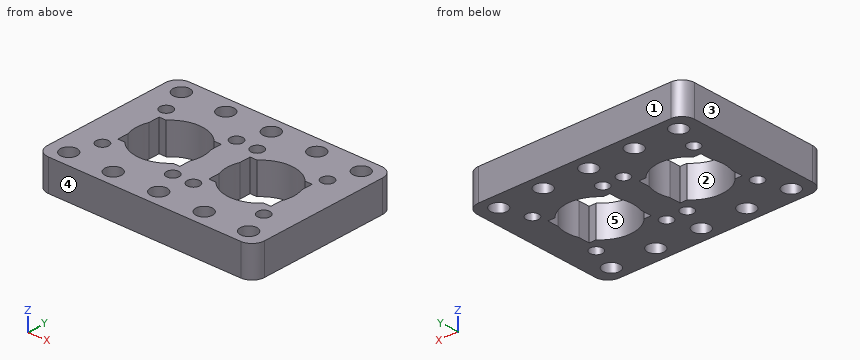
Autodesk Inventor part; units mm, degrees
ref_plane "YZ Plane" through (0, 0, 0) normal (1, 0, 0) x (0, 1, 0)
ref_plane "XZ Plane" through (0, 0, 0) normal (0, 1, 0) x (-1, 0, 0)
ref_plane "XY Plane" through (0, 0, 0) normal (0, 0, 1) x (1, 0, 0)
sketch "Sketch1" plane through (0, 0, 0) normal (0, 0, 1) x (1, 0, 0)
  line L0 (-22, 0) -> (22, 0) construction
  circle A0 centre (-22, 0) radius 16
  circle A1 centre (22, 0) radius 16
  line L1 (43.5, -30) -> (-43.5, -30) construction
  line L2 (-43.5, -30) -> (-43.5, 30) construction
  line L3 (-43.5, 30) -> (43.5, 30) construction
  line L4 (43.5, 30) -> (43.5, -30) construction
  line L5 (43.5, -30) -> (-43.5, 30) construction
  line L6 (-43.5, -30) -> (43.5, 30) construction
  circle A2 centre (-43.5, 30) radius 4
  circle A3 centre (0, 30) radius 4
  circle A4 centre (43.5, 30) radius 4
  circle A5 centre (43.5, -30) radius 4
  circle A6 centre (-43.5, -30) radius 4
  circle A7 centre (0, -30) radius 4
  line L7 (-52.5, -37.5) -> (52.5, -37.5)
  line L8 (52.5, -37.5) -> (52.5, 37.5)
  line L9 (52.5, 37.5) -> (-52.5, 37.5)
  line L10 (-52.5, 37.5) -> (-52.5, -37.5)
  line L11 (-52.5, -37.5) -> (52.5, 37.5) construction
  line L12 (52.5, -37.5) -> (-52.5, 37.5) construction
  line L13 (-5, -17) -> (-39, -17) construction
  line L14 (-39, -17) -> (-39, 17) construction
  line L15 (-39, 17) -> (-5, 17) construction
  line L16 (-5, 17) -> (-5, -17) construction
  line L17 (-5, -17) -> (-39, 17) construction
  line L18 (-39, -17) -> (-5, 17) construction
  line L19 (39, -17) -> (5, -17) construction
  line L20 (5, -17) -> (5, 17) construction
  line L21 (5, 17) -> (39, 17) construction
  line L22 (39, 17) -> (39, -17) construction
  line L23 (39, -17) -> (5, 17) construction
  line L24 (5, -17) -> (39, 17) construction
  circle A8 centre (-39, 17) radius 3
  circle A9 centre (-39, -17) radius 3
  circle A10 centre (-5, -17) radius 3
  circle A11 centre (-5, 17) radius 3
  circle A12 centre (5, 17) radius 3
  circle A13 centre (5, -17) radius 3
  circle A14 centre (39, -17) radius 3
  circle A15 centre (39, 17) radius 3
  point P0 (0, 0)
  point P1 (0, 0)
  dimension "d0" = 60
  dimension "d1" = 87
  dimension "d2" = 44
  dimension "d3" = 32
  dimension "d4" = 8
  dimension "d5" = 105
  dimension "d6" = 75
  dimension "d10" = 34
  dimension "d11" = 6
extrude "Extrusion1" add sketch "Sketch1" along normal blind 15
fillet "Fillet1" radius 6 4 edges at (-52.5, 37.5, 7.5) (52.5, 37.5, 7.5) (52.5, -37.5, 7.5) (-52.5, -37.5, 7.5)
sketch "Sketch2" plane through (0, 0, 15) normal (0, 0, 1) x (1, 0, 0)
  circle A0 centre (22, 0) radius 16
  circle A1 centre (-22, 0) radius 16
  line L0 (37, -11) -> (7, -11)
  line L1 (7, -11) -> (7, 11)
  line L2 (7, 11) -> (37, 11)
  line L3 (37, 11) -> (37, -11)
  line L4 (37, -11) -> (7, 11) construction
  line L5 (7, -11) -> (37, 11) construction
  line L6 (-37, -11) -> (-7, -11)
  line L7 (-7, -11) -> (-7, 11)
  line L8 (-7, 11) -> (-37, 11)
  line L9 (-37, 11) -> (-37, -11)
  line L10 (-37, -11) -> (-7, 11) construction
  line L11 (-7, -11) -> (-37, 11) construction
  point P0 (0, 0)
  dimension "d12" = 22
  dimension "d13" = 30
extrude "Extrusion2" cut sketch "Sketch2" against normal through all contours L3 A0 L0 L1 L2 | A0 L2 L3 | L3 L0 A0 | A0 L1 L2 | L0 L1 A0 | L7 A1 L6 L9 L8 | A1 L8 L7 | L7 L6 A1 | A1 L9 L8 | L6 L9 A1
sketch "Sketch3" plane through (0, 0, 15) normal (0, 0, 1) x (1, 0, 0)
  arc A0 (-10.381, 11) -> (-33.619, 11) centre (-22, 0) ccw construction
  arc A1 (33.619, 11) -> (10.381, 11) centre (22, 0) ccw construction
  line L0 (-22, -30) -> (22, -30) construction
  line L1 (22, -30) -> (22, 30) construction
  line L2 (22, 30) -> (-22, 30) construction
  line L3 (-22, 30) -> (-22, -30) construction
  line L4 (-22, -30) -> (22, 30) construction
  line L5 (22, -30) -> (-22, 30) construction
  circle A2 centre (0, 30) radius 4 construction
  circle A3 centre (-22, 30) radius 4
  circle A4 centre (22, 30) radius 4
  circle A5 centre (22, -30) radius 4
  circle A6 centre (-22, -30) radius 4
  point P0 (0, 0)
  dimension "d16" = 8
extrude "Extrusion3" cut sketch "Sketch3" against normal through all
properties part number "cylinder frame"
The model under review builds one solid part; all positions refer to its coordinate system, in mm. Face numbers are marked on the shaded views. A direction names the side the tool comes from. Coordinates: 2 decimals unless noted, no trailing zeros. Order: outer loops, then holes, each group sorted by start corner. A loop starts at its lowest first (then second) coordinate and runs counter-clockwise, first axis right, second up. Notation, with made-up numbers: (68, 76.5) -> (75, 76.5) arc R23 ccw to (75, 111.5) -> close; hole circle Ø7 at (70.25, -7). An arc over 180 degrees is marked (long way). Answer in a Markdown table with one row per item.
(1) Consider section A-A (y = -9). Write out the cut boundary in (x, z).
Answers:
| item | result |
|---|---|
| outline | (-52.5, 0) -> (-37, 0) -> (-37, 15) -> (-52.5, 15) -> close; (-7, 0) -> (7, 0) -> (7, 15) -> (-7, 15) -> close; (37, 0) -> (52.5, 0) -> (52.5, 15) -> (37, 15) -> close |
(2) Consider section B-B (x = 0). Write out the cut boundary in (y, z), plus the area to 3 significant figures.
Answers:
| item | result |
|---|---|
| outline | (-37.5, 0) -> (-34, 0) -> (-34, 15) -> (-37.5, 15) -> close; (-26, 0) -> (26, 0) -> (26, 15) -> (-26, 15) -> close; (34, 0) -> (37.5, 0) -> (37.5, 15) -> (34, 15) -> close |
| area | 885 mm² |
(3) The part is to be moulded in two halves that separate along X. For the marked faces 3, 4 and 5, say which applies: +X half, -X half, draft (parallel to the pull), parting line (faces both ways), or undercut.
Answers:
| item | result |
|---|---|
| face 3 | -X half |
| face 4 | draft |
| face 5 | undercut |
(4) Consider section D-D (x = 22). Write out the cut boundary in (y, z).
Answers:
| item | result |
|---|---|
| outline | (-37.5, 0) -> (-34, 0) -> (-34, 15) -> (-37.5, 15) -> close; (-26, 0) -> (-16, 0) -> (-16, 15) -> (-26, 15) -> close; (16, 0) -> (26, 0) -> (26, 15) -> (16, 15) -> close; (34, 0) -> (37.5, 0) -> (37.5, 15) -> (34, 15) -> close |
(5) Machinability: for the marked faces 1 and 2, which of the approach directions +Z, -Z, +X, -X, +Y, -Y give a long, thin tool a straight path to every point of the face, cutting with its end or side? Answer none if there is none.
Answers:
| item | result |
|---|---|
| face 1 | +Z, -Z, +X, -X, +Y |
| face 2 | +Z, -Z |
(6) Consider section C-C (y = -30). Write out the cut boundary in (x, z).
Answers:
| item | result |
|---|---|
| outline | (-52.5, 0) -> (-47.5, 0) -> (-47.5, 15) -> (-52.5, 15) -> close; (-39.5, 0) -> (-26, 0) -> (-26, 15) -> (-39.5, 15) -> close; (-18, 0) -> (-4, 0) -> (-4, 15) -> (-18, 15) -> close; (4, 0) -> (18, 0) -> (18, 15) -> (4, 15) -> close; (26, 0) -> (39.5, 0) -> (39.5, 15) -> (26, 15) -> close; (47.5, 0) -> (52.5, 0) -> (52.5, 15) -> (47.5, 15) -> close |
(7) Wall thickness on line 1 along X through (y, z) = (-7, 4.5); line 2 along Y through (x, z) = (-39, 5.5); line 3 along Y through (x, z) = (22, 7.75): over which ranges is each line inside the solid? List them lowest first.
Answers:
| item | result |
|---|---|
| line 1 | -52.5 to -37, -7 to 7, 37 to 52.5 |
| line 2 | -37.5 to -20, -14 to 14, 20 to 37.5 |
| line 3 | -37.5 to -34, -26 to -16, 16 to 26, 34 to 37.5 |
